Source: CAD feature listing. Evaluate the final solid. Frame: model axes, mm. A direction names the side the tool comes from. Give positions to 0.01 mm unless a question says otherwise; leave off trailing zeros. Order: outer loops, then holes, each group sorted by start corner. A loop starts at its lowest first (then second) coordinate and runs counter-clockwise, first axis right, second up. Notation, with made-up numbers: M -3.75,85.5 L 38.25,85.5 A5 cw 38.25,92.5 Z; hole C 21,-24.5 d4. An arc over 180 degrees is marked long. Answer in a Markdown table with one row per item. Add a question column.
(1) Section query C-C, the plane z = 6. Return loops of the section in (x, y), plus the area to 3 significant figures.
(2) Section query D-D, the plane z = 7.75. Return loops of the section in (x, y).
(3) Pin query (flat end, axial travel): P1, Ø4, axis at x = 1, y = 0, coming from the -Z side; P2, Ø1.5, axis at y = -1, z = 2.5, coming from the +X side; P3, Ø1.5, axis at x = -2, z = 2, coming from the +Y side; P4, Ø1, axis at x = -1.5, z = 8.5, coming from the -Y side. Return the tip coordinate at first contact, or that it passes through.
(4) Section query B-B, the plane y = 3. Return loops of the section in (x, z), plus the area to 4 significant figures.
(5) Section query A-A, the plane x = 0. Return loops of the section in (y, z), plus the area to 4 significant figures.
(6) Set-up query: faces 1 (the face through (-0.89, -2.45, 0)), 2 (the face through (1, 4, 4.5)). Return all of +Z, -Z, +X, -X, +Y, -Y with unobstructed straight access to the full face (end or side cutting, diameter ignored); none if empty.
(7) Mould query, pull axis Y, two halves, no side actions, for faces 3 (the face through (0, 0, 7)), 4 (the face through (0, 0, 9.5)), 5 (the face through (-0.5, -2.4, 3.5)), 6 (the face through (-1.08, -4.88, 6.96)). Classes: pulls with the +Y half, pulls with the -Y half, needs draft (parallel to the pull), parting line crosses it, or undercut.
(8) Material intervals for line 1 along Y through (x, z) = (0, 2); line 2 along Y through (x, z) = (0, 5); line 3 along Z through (x, y) = (-2, -0.75), sorted ascending.
from build123d import *

# Parameters (mm, degrees)
F0_R     = 3.75
F0_R_2   = 2.45
F1_DEPTH = 4.5
F2_R     = 5
F3_DEPTH = 5
F4_R     = 2.45
F5_DEPTH = 2.5


with BuildPart() as f1:
    # F0 (on Top) → F1 (new body)
    with BuildSketch(Plane.XY):
        Circle(F0_R)
        Circle(F0_R_2, mode=Mode.SUBTRACT)
    extrude(amount=F1_DEPTH)

    # F2 (on face) → F3 (join)
    with BuildSketch(Plane.XY.offset(4.5)):
        Circle(F2_R)
    extrude(amount=F3_DEPTH)

    # F4 (on face) → F5 (cut)
    with BuildSketch(Plane(origin=(0, 0, 4.5), x_dir=(1, 0, 0), z_dir=(0, 0, -1))):
        Circle(F4_R)
    extrude(amount=-F5_DEPTH, mode=Mode.SUBTRACT)


solid = f1.part
Values follow:
| question | item | result |
|---|---|---|
| 1 | outline | C 0,0 d10; hole C 0,0 d4.9 |
| 1 | area | 59.7 mm² |
| 2 | outline | C 0,0 d10 |
| 3 | P1 | stops at z = 0 |
| 3 | P2 | stops at x = 3.74 |
| 3 | P3 | stops at y = 3.54 |
| 3 | P4 | stops at y = -4.9 |
| 4 | outline | M -4,4.5 L -2.25,4.5 L -2.25,0 L 2.25,0 L 2.25,4.5 L 4,4.5 L 4,9.5 L -4,9.5 Z |
| 4 | area | 60.25 mm² |
| 5 | outline | M -5,4.5 L -3.75,4.5 L -3.75,0 L -2.45,0 L -2.45,7 L 2.45,7 L 2.45,0 L 3.75,0 L 3.75,4.5 L 5,4.5 L 5,9.5 L -5,9.5 Z |
| 5 | area | 49.45 mm² |
| 6 | face 1 | -Z, +X, -X, +Y, -Y |
| 6 | face 2 | -Z |
| 7 | face 3 | undercut |
| 7 | face 4 | needs draft |
| 7 | face 5 | undercut |
| 7 | face 6 | parting line crosses it |
| 8 | line 1 | y = -3.75 to -2.45, 2.45 to 3.75 |
| 8 | line 2 | y = -5 to -2.45, 2.45 to 5 |
| 8 | line 3 | z = 7 to 9.5 |
